Part model, mm, in its own coordinate system. Face numbers are marked on the shaded views. Round coordinates to 2 decimals unless told otherwise and drop trailing zeros. Loops run counter-clockwise (first coordinate to the right, second up) from the corner with the lowest first, then second, coordinate; pieces in that order, holes last. Notation, with made-up numbers: (1.5, 22.5) - (17.5, 22.5) arc R34 cw to (17.5, 57.5) - close; hole circle Ø3 at (53, -23.75). An arc over 180 degrees is marked (long way). Put each result on its own line as item: value.
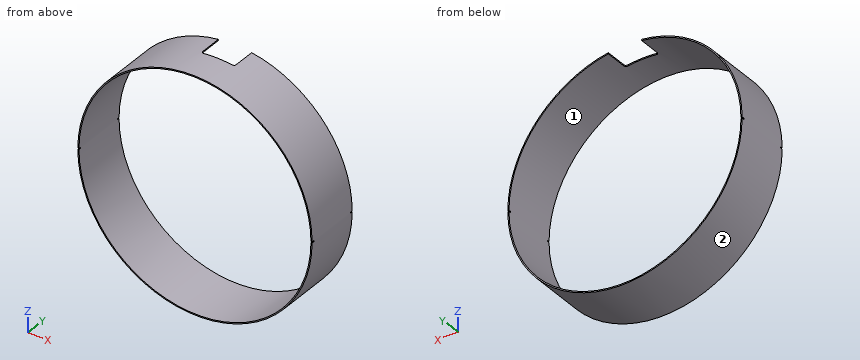
from build123d import *

# Parameters (mm, degrees)
SKETCH_1_R               = 50.3
SKETCH_1_R_2             = 49.8
EXTRUDE_1_DEPTH          = 24
CUT_EXTRUDE_1_DEPTH      = 52
CUT_EXTRUDE_2_DEPTH      = 52
CUT_EXTRUDE_2_DEPTH_BACK = 52
FILLET_1_R               = 1


with BuildPart() as part:
    # Эскиз1 → Бобышка-Вытянуть1 (new body)
    with BuildSketch(Plane(origin=(0, 0, 0), x_dir=(1, 0, 0), z_dir=(0, 1, 0))):
        with Locations(Location((0, 0, 0), (0, 0, 270))):
            Circle(SKETCH_1_R)
        with Locations(Location((0, 0, 0), (0, 0, 270))):
            Circle(SKETCH_1_R_2, mode=Mode.SUBTRACT)
    extrude(amount=EXTRUDE_1_DEPTH)

    # Эскиз2 → Вырез-Вытянуть1 (cut)
    with BuildSketch(Plane.XY):
        Polygon((-7.130200452, 13.65), (-7.158835795, 24), (7.158835795, 24), (7.130200452, 13.65), align=None)
    extrude(amount=CUT_EXTRUDE_1_DEPTH, mode=Mode.SUBTRACT)

    # Эскиз3 → Вырез-Вытянуть2 (cut, two sides: drawn at the far end of the back side and taken through both)
    with BuildSketch(Plane(origin=(0, 0, 0), x_dir=(0, 0, -1), z_dir=(1, 0, 0)).offset(-CUT_EXTRUDE_2_DEPTH_BACK)):
        Polygon((0, 24), (0.25, 24), (0.25, 23), (-0.25, 23), (-0.25, 24), align=None)
        Polygon((0.25, 1), (0.25, 0), (0, 0), (-0.25, 0), (-0.25, 1), align=None)
    extrude(amount=CUT_EXTRUDE_2_DEPTH + CUT_EXTRUDE_2_DEPTH_BACK, mode=Mode.SUBTRACT)

    # Скругление1
    fillet_1_edges = [part.edges().sort_by_distance(p)[0] for p in [
        (7.130200452, 13.65, 49.539493808),
        (-7.130200452, 13.65, 49.539493808),
    ]]
    fillet(fillet_1_edges, radius=FILLET_1_R)


solid = part.part
1. Pin check, flat tips, straight feed: P1, Ø1, axis at x = 35.5, y = 19, coming from the -Z side; P2, Ø6, axis at x = 35.5, y = 20, coming from the -Z side; P3, Ø1.5, axis at x = 9.5, y = 11, coming from the +Z side. Stop position of each tip, or through.
A:
P1: stops at z = -36.13
P2: stops at z = -38.39
P3: stops at z = 49.53
2. Band-saw the part on C-C (y = 8.75). List the corners of the cut face in (x, z), plus the area to 3 significant figures.
A:
outline: circle Ø100.6 at (0, 0); hole circle Ø99.6 at (0, 0)
area: 157 mm²
3. Probe line 1 along X through (y, z) = (11.5, 0); line 2 along Z through (x, y) = (45, 19.75). List the from-to ranges inside material, lowest first. Write a range as [from, to].
A:
line 1: x = [-50.3, -49.8], [49.8, 50.3]
line 2: z = [-22.47, -21.33], [21.33, 22.47]
4. Band-saw the part on D-D (y = 20). List the corners of the cut face in (x, z).
A:
outline: (-7.15, 49.28) - (-7.15, 49.79) arc R50.3 ccw (long way) to (7.15, 49.79) - (7.15, 49.28) arc R49.8 cw (long way) to start
5. Two-plate mould, pull along Z, no slides. Class the marked faces 1 and 2: pulls with the +Z half, pulls with the -Z half, needs draft (parallel to the pull), parting line crosses it, or undercut.
A:
face 1: undercut
face 2: parting line crosses it
6. Band-saw the part on B-B (z = 24.5). List the corners of the cut face in (x, y).
A:
outline: (-43.93, 0) - (-43.36, 0) - (-43.36, 24) - (-43.93, 24) - close; (43.36, 0) - (43.93, 0) - (43.93, 24) - (43.36, 24) - close
7. Band-saw the part on A-A (x = 0). List the corners of the cut face in (y, z), plus the area to 3 significant figures.
A:
outline: (0, -50.3) - (24, -50.3) - (24, -49.8) - (0, -49.8) - close; (0, 49.8) - (13.65, 49.8) - (13.65, 50.3) - (0, 50.3) - close
area: 18.8 mm²
